```python
from build123d import *

# Parameters (mm, degrees)
M5_CLEARANCE_HOLE1_D = 5.5
FILLET1_R            = 0.2
CHAMFER1_SIZE        = 0.5


with BuildPart() as part:
    # Sketch1 → Revolve1 (revolve)
    with BuildSketch(Plane.XY, mode=Mode.PRIVATE) as revolve1_sk:
        Polygon((14, -3), (14, 12.15), (12, 12.15), (12, 15.15), (19, 15.15), (19, 0), (39, 0), (39, -3), align=None)
    revolve(revolve1_sk.sketch.rotate(Axis((0, 17.954019247, 0), (0, -1, 0)), 90), axis=Axis((0, 17.954019247, 0), (0, -1, 0)))

    # M5 Clearance Hole1 (through all)
    with Locations(Plane(origin=(0, 0, 0), x_dir=(1, 0, 0), z_dir=(0, 1, 0))):
        with Locations((0, 29), (29, 0), (0, -29), (-29, 0)):
            Hole(M5_CLEARANCE_HOLE1_D / 2)

    # Fillet1
    fillet1_edges = [part.edges().sort_by_distance(p)[0] for p in [
        (0, 0, -19),
        (0, 12.15, -14),
    ]]
    fillet(fillet1_edges, radius=FILLET1_R)

    # Chamfer1
    chamfer1_edges = [part.edges().sort_by_distance(p)[0] for p in [
        (0, 12.15, -12),
        (0, 15.15, -12),
        (0, 15.15, -19),
        (0, 0, -39),
        (0, -3, -39),
        (0, -3, -14),
    ]]
    chamfer(chamfer1_edges, length=CHAMFER1_SIZE)

    # Sketch14 → Groove for BS 3673 P4 - B028M, Internal Circlip1 (revolve, cut)
    with BuildSketch(Plane(origin=(0, 17.954019247, 0), x_dir=(0, 0, 1), z_dir=(-1, 0, 0))):
        with BuildLine():
            Line((14.57, -14.104019247), (12.6, -14.104019247))
            Line((12.6, -14.104019247), (12.6, -12.804019247))
            Line((12.6, -12.804019247), (14.57, -12.804019247))
            ThreePointArc((14.57, -12.804019247), (14.661923882, -12.842095365), (14.7, -12.934019247))
            Line((14.7, -12.934019247), (14.7, -13.974019247))
            ThreePointArc((14.7, -13.974019247), (14.661923882, -14.065943128), (14.57, -14.104019247))
        make_face()
    revolve(axis=Axis((0, -32.045980753, 0), (0, 1, 0)), mode=Mode.SUBTRACT)


solid = part.part
```
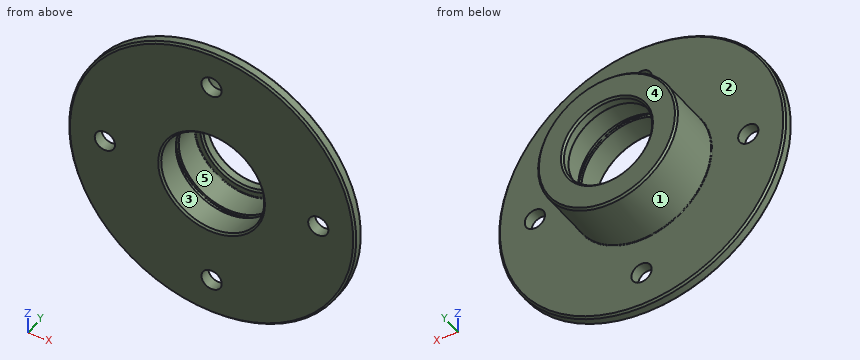
CAD build for the part. Positions are in the model's coordinates, mm. Face numbers are marked on the shaded views. A direction names the side the tool comes from. Coordinates: 2 decimals unless noted, no trailing zeros. Write each loop counter-clockwise with the first axis right and the second up, starting at its lowest first coordinate (ties: lowest second). Pieces come first, ordered by that corner, then holes.
(1) Flat gauge pins, fed straight in: pin 1 (2 mm diameter, centred on x = -4, y = -0.5, fed in from +Z); pin 2 (5 mm diameter, centred on x = -0.5, y = 12, fed in from -Z); pin 3 (3 mm diameter, centred on y = 9, z = 17, fed in from -X). Where does each tip first touch, or does it go through?
(2) Cut at B-B, the plane y = 6.25. List the corners of the cut face in (x, z), and give its area (3 significant figures).
(3) Two-plate mould, pull along X, no slides. Class the marked faces 1, 2 and 3: +X half, -X half, draft (parallel to the pull), parting line (faces both ways), or undercut.
(4) 3-axis set-ups, long thin cutter, end or side, ignore diameter. For the marked faces 4 and 5: which of +Z, -Z, +X, -X, +Y, -Y reach the whole face in a straight line?
(5) Drill centre lines: probe 1 along X at (y, z) = (4.6, 0); probe 2 along X at (y, z) = (0.5, 0); probe 3 along Y at (x, z) = (-29, -23). Where is each one in solid material? Low to high.
(6) Cut at A-A, the plane x = 0. Count the separate pieces of the cut face and the enclosed holes in it, and give its area (3 significant figures).
Geometry says:
1. pin 1: stops at z = 38.88
1. pin 2: stops at z = -19
1. pin 3: stops at x = -10.99
2. outline: circle Ø38 at (0, 0); hole circle Ø28 at (0, 0)
2. area: 518 mm2
3. face 1: parting line
3. face 2: draft
3. face 3: undercut
4. face 4: +Z, -Z, +X, -X, +Y
4. face 5: -Y
5. probe 1: x = -19 to -14.7, 14.7 to 19
5. probe 2: x = -19 to -14, 14 to 19
5. probe 3: y = -3 to 0
6. separate pieces: 4
6. enclosed holes: 0
6. area: 277 mm2
